Autodesk Inventor part; units mm, degrees
ref_plane "YZ Plane" through (0, 0, 0) normal (1, 0, 0) x (0, 1, 0)
ref_plane "XZ Plane" through (0, 0, 0) normal (0, 1, 0) x (-1, 0, 0)
ref_plane "XY Plane" through (0, 0, 0) normal (0, 0, 1) x (1, 0, 0)
sketch "Sketch1" plane through (0, 0, 0) normal (0, 1, 0) x (-1, 0, 0)
  line L0 (0, 0) -> (0, -317.5)
  line L1 (0, -317.5) -> (33.528, -317.5)
  line L2 (33.528, -317.5) -> (33.528, 0)
  line L3 (33.528, 0) -> (0, 0)
  dimension "d0" = 317.5
  dimension "d1" = 33.528
extrude "Extrusion1" add sketch "Sketch1" along normal blind 1.778
sketch "Sketch2" plane through (0, 1.778, 0) normal (0, 1, 0) x (1, 0, 0)
  line L0 (-33.528, 0) -> (0, 0)
  line L1 (-33.528, 0) -> (-31.75, 0)
  line L2 (-31.75, 0) -> (-31.75, 317.5)
  line L3 (-33.528, 317.5) -> (-33.528, 0)
  line L4 (-31.75, 317.5) -> (-33.528, 317.5)
  line L5 (-33.528, 317.5) -> (-33.528, 0)
  dimension "d4" = 1.778
extrude "Extrusion2" add sketch "Sketch2" along normal blind 31.75
properties part number "Long Boi" material "Steel, Alloy"
The model under review builds one solid part; all positions refer to its coordinate system, in mm. A direction names the side the tool comes from. Give positions to 0.01 mm unless a question says otherwise; leave off trailing zeros. Write each loop counter-clockwise with the first axis right and the second up, starting at its lowest first coordinate (ties: lowest second). Pieces come first, ordered by that corner, then holes. Notation, with made-up numbers: M 78,40 L 100,40 A22 ccw 100,66 Z; hole C -34.5,36.5 d4. An arc over 180 degrees is marked long. One line per question, with ' | ' between items. Start each with the question number.
Item 1: We need section C-C on x = -13.5. Write out the cut boundary in (y, z), plus the area to 3 significant figures.
Item 2: For pin 1 (2 mm diameter, centred on x = -15, z = -188.5, fed in from -Y); pin 2 (4 mm diameter, centred on x = -9.5, z = -96.5, fed in from +Y); pin 3 (1 mm diameter, centred on y = 26, z = -280.5, fed in from +X), all flat-tipped, find the tip position at first contact; note any pin that passes through.
Item 3: We need section B-B on y = 16. Write out the cut boundary in (x, z), plus the area to 3 significant figures.
Item 4: For faces 1 (the flat face through (-33.528, 17, -161)), 2 (the flat face through (-31.75, 17, -157)), list the 3-axis set-ups (+Z, -Z, +X, -X, +Y, -Y) from which the entire face can be reached by the end or side of a thin tool; tool diameter is ignored.
Item 5: We need section A-A on z = -22. Write out the cut boundary in (x, y).
Item 6: Wall thickness on line 1 (Y direction, x = -23, z = -99.5); line 2 (X direction, y = 27, z = -45): over which ranges is each line inside the solid? List them lowest first. Write a range as from..to.
Results found:
1) outline: M 0,-317.5 L 1.78,-317.5 L 1.78,0 L 0,0 Z | area: 565 mm2
2) pin 1: stops at y = 0 | pin 2: stops at y = 1.78 | pin 3: stops at x = -31.75
3) outline: M -33.53,-317.5 L -31.75,-317.5 L -31.75,0 L -33.53,0 Z | area: 565 mm2
4) face 1: +Z, -Z, -X, +Y, -Y | face 2: +Z, -Z, +X, +Y
5) outline: M -33.53,0 L 0,0 L 0,1.78 L -31.75,1.78 L -31.75,33.53 L -33.53,33.53 Z
6) line 1: y = 0..1.78 | line 2: x = -33.53..-31.75
